from build123d import *

# Parameters (mm, degrees)
EXTRUDE_473_DEPTH = 5
FILLET_R_R        = 10


with BuildPart() as part:
    # ｽｹｯﾁ1 → Extrude 473 (new, symmetric)
    with BuildSketch(Plane(origin=(0, 0, 0), x_dir=(1, 0, 0), z_dir=(0, 1, 0))):
        Polygon((-166, 36), (-76, 36), (-76, 38), (100, 38), (100, -38), (-76, -38), (-76, -36), (-166, -36), align=None)
    extrude(amount=EXTRUDE_473_DEPTH, both=True)

    # 外周 角R
    fillet_r_edges = [part.edges().sort_by_distance(p)[0] for p in [
        (-166, 0, -36),
        (100, 0, -38),
        (100, 0, 38),
        (-166, 0, 36),
    ]]
    fillet(fillet_r_edges, radius=FILLET_R_R)


solid = part.part
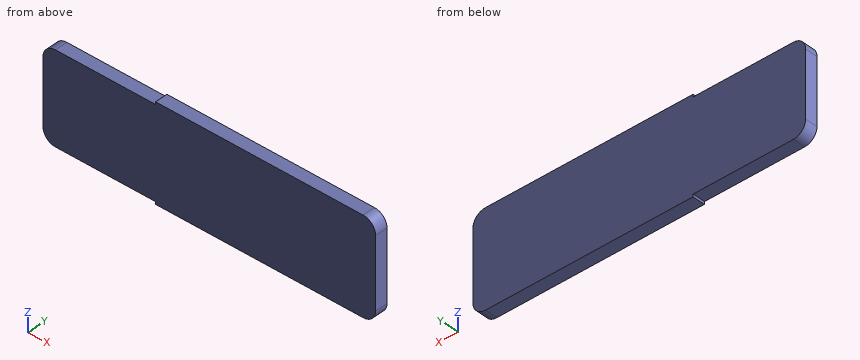
Build history of the part. All positions in model axes, mm. Give positions to 0.01 mm unless a question says otherwise; leave off trailing zeros. Order: outer loops, then holes, each group sorted by start corner. A loop starts at its lowest first (then second) coordinate and runs counter-clockwise, first axis right, second up. Notation, with made-up numbers: M 75,76.25 L 120,76.25 A17 ccw 120,101.25 Z; hole C -19,-2.5 d5. An arc over 180 degrees is marked long. Put each result on its own line as item: value.
Item 1: Cut at B-B on x = -78.5. Write the cut outline in (y, z), then the cut area to 3 significant figures.
Results are:
outline: M -5,-36 L 5,-36 L 5,36 L -5,36 Z
area: 720 mm2
Item 2: Cut at A-A on y = 1.5. Write the cut outline in (x, z), then the cut area to 3 significant figures.
Results are:
outline: M -166,-26 A10 ccw -156,-36 L -76,-36 L -76,-38 L 90,-38 A10 ccw 100,-28 L 100,28 A10 ccw 90,38 L -76,38 L -76,36 L -156,36 A10 ccw -166,26 Z
area: 19,800 mm2
Item 3: Wall check: probe 1 along X at (y, z) = (2.5, 27); probe 2 along Z at (x, y) = (-86.5, 4.75); probe 3 along X at (y, z) = (2, 26.5). Give the ranges that are in metal, low to high.
Results are:
probe 1: -165.95 to 100
probe 2: -36 to 36
probe 3: -165.99 to 100
Item 4: Drop flat-ended pins along their axis: pin 1 Ø1.6 at (y, z) = (-1, -37.5) entering from -X; pin 2 Ø3 at (x, y) = (-97, 2) entering from +Z. Give the stop position or say it passes through.
Results are:
pin 1: x = -76
pin 2: z = 36
